Drawing for the job (mm, zero at the part's lowest x, y, z). Round coordinates to 2 decimals unless told otherwise and drop trailing zeros. Write each loop counter-clockwise with the first axis right and the second up, starting at its lowest first coordinate (ties: lowest second). Pieces come first, ordered by that corner, then holes. Notation, with made-up numbers: M -32,89 L -10,89 A27 ccw -10,128 Z; hole C 75.5,-17 d7. An arc over 180 degrees is marked long. Use a Markdown table: item, result. Add a question column.
1) Wall check: probe 1 along Z at (x, y) = (34.5, 1.7); probe 2 along X at (y, z) = (0.75, 40); probe 3 along X at (y, z) = (2.55, 9). Give the ranges that are in metal, low to high.
2) Slice it at A-A on x = 26.5. Write the cut outline in (y, z).
3) Drop flat-ended pins along their axis: P1, Ø0.9, axis at x = 129, y = 2, coming from the -Z side; P2, Ø0.6, axis at y = 2, z = 40, coming from the -X side; P3, Ø0.9, axis at x = 137.5, y = 2, coming from the -Z side; P4, Ø1.5, axis at y = 1.5, z = 41, coming from the +X side. Give the stop position or say it passes through.
4) Slice it at C-C on y = 0.6. Give the number of separate pieces and of enclosed holes in the cut face, plus the area to 3 significant figures.
5) Slice it at B-B on z = 67.5. Write the cut outline in (x, y), plus the area to 4 significant figures.
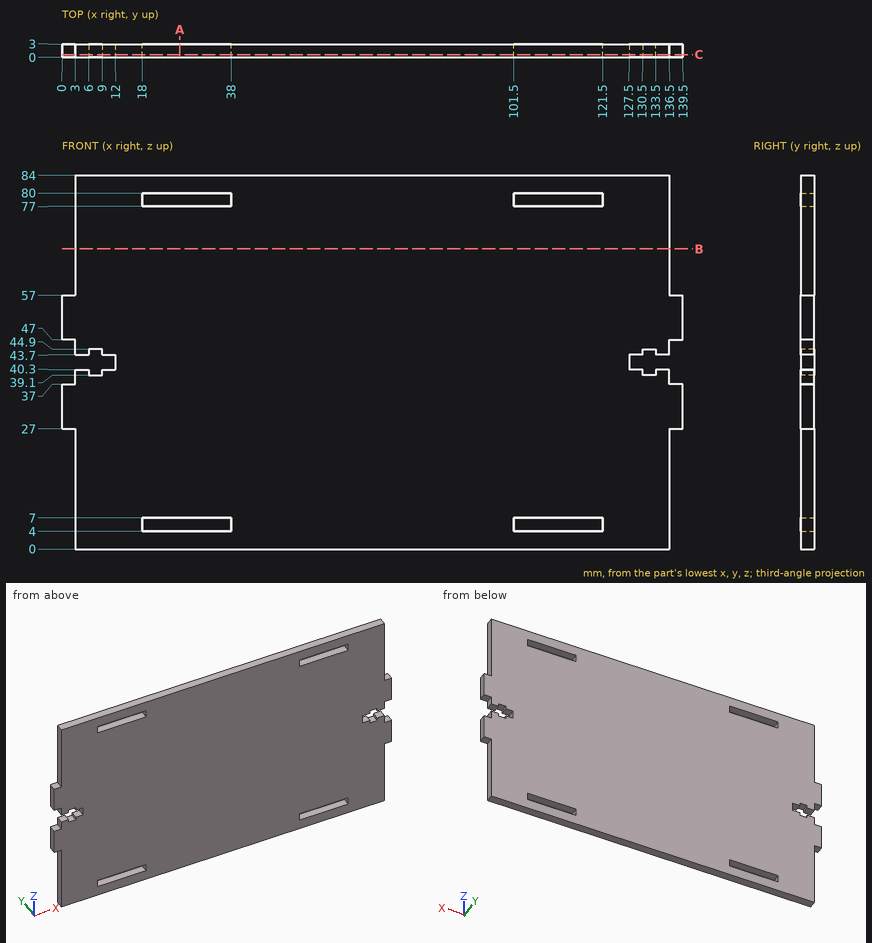
Entries:
| question | item | result |
|---|---|---|
| 1 | probe 1 | z = 0 to 4, 7 to 77, 80 to 84 |
| 1 | probe 2 | x = 3 to 6, 9 to 130.5, 133.5 to 136.5 |
| 1 | probe 3 | x = 3 to 136.5 |
| 2 | outline | M 0,0 L 3,0 L 3,4 L 0,4 Z; M 0,7 L 3,7 L 3,77 L 0,77 Z; M 0,80 L 3,80 L 3,84 L 0,84 Z |
| 3 | P1 | stops at z = 0 |
| 3 | P2 | stops at x = 3 |
| 3 | P3 | stops at z = 27 |
| 3 | P4 | stops at x = 136.5 |
| 4 | separate pieces | 1 |
| 4 | enclosed holes | 4 |
| 4 | area | 11,000 mm^2 |
| 5 | outline | M 3,0 L 136.5,0 L 136.5,3 L 3,3 Z |
| 5 | area | 400.5 mm^2 |
